Autodesk Inventor part; units mm, degrees
ref_plane "YZ Plane" through (0, 0, 0) normal (1, 0, 0) x (0, 1, 0)
ref_plane "XZ Plane" through (0, 0, 0) normal (0, 1, 0) x (-1, 0, 0)
ref_plane "XY Plane" through (0, 0, 0) normal (0, 0, 1) x (1, 0, 0)
sketch "Sketch1" plane through (0, 0, 0) normal (0, 0, 1) x (1, 0, 0)
  circle A0 centre (0, 0) radius 5
  circle A1 centre (0, 0) radius 2.5
  dimension "d0" = 10
  dimension "d1" = 5
extrude "Extrusion1" add sketch "Sketch1" along normal mid plane 4.2
sketch "Sketch2" plane through (0, 0, 2.1) normal (0, 0, 1) x (1, 0, 0)
  circle A0 centre (0, 0) radius 2.5
  circle A1 centre (0, 0) radius 5
  circle A2 centre (0, 0) radius 4.5
  circle A3 centre (0, 0) radius 4.1
  circle A4 centre (0, 0) radius 2.95
  circle A5 centre (0, 0) radius 3.35
  dimension "d4" = 0.5
  dimension "d5" = 0.4
  dimension "d6" = 0.75
  dimension "d7" = 0.4
extrude "Extrusion2" cut sketch "Sketch2" against normal blind 0.5 contours A2 | A5
fillet "Fillet1" radius 0.15 2 edges at (-4.1, 0, 2.1) (-3.35, 0, 2.1)
mirror "Mirror1" about plane through (0, 0, 0) normal (0, 0, 1) of "Extrusion2"
fillet "Fillet2" radius 0.15 2 edges at (-4.1, 0, -2.1) (-3.35, 0, -2.1)
properties part number "Mini Bearing" material "Steel"
Can you work these out from the model? Positions are in its coordinate system, mm. A direction names the side the tool comes from. Give positions to 0.01 mm unless a question says otherwise; leave off trailing zeros. Loops run counter-clockwise (first coordinate to the right, second up) from the corner with the lowest first, then second, coordinate; pieces in that order, holes last. Notation, with made-up numbers: (-32.75, -26.75) -> (-5.75, -26.75) arc R14 ccw to (-5.75, -7.75) -> close; hole circle Ø8 at (33.5, 14). An arc over 180 degrees is marked (long way). Return JSON: item names as keys, results as strings.
Q1. I want a section at A-A, the plane z = -0.45. List the corners of the cut face in (x, y) for me.
Checks:
{"outline": "circle Ø10 at (0, 0); hole circle Ø5 at (0, 0)"}
Q2. On a 3-axis mill with a long thin cutter (end or side, diameter ignored), from which of +Z, -Z, +X, -X, +Y, -Y can I reach the whole of each face in a straight line? I mean faces 1 (the face through (-0.54, -2.44, 0.03)), 2 (the face through (-0.534, 4.065, 1.777)), 3 (the face through (-1, -3, -1.6)). Say none if no direction works.
Checks:
{"face 1": "+Z, -Z", "face 2": "+Z", "face 3": "-Z"}
Q3. For pin 1 Ø1 at (x, z) = (-1, 1) entering from -Y; pin 2 Ø4.5 at (x, y) = (0, 0) entering from -Z, each with a flat end and sliding along its axis, tell me the tip position at first contact or that it passes through.
Checks:
{"pin 1": "stops at y = -4.97", "pin 2": "passes through"}
Q4. I need wall thicknesses on probe 1 along Y at (x, z) = (0, 1.8); probe 2 along X at (y, z) = (1.5, -1.7); probe 3 along Z at (x, y) = (-2.25, 3.5). Which ranges of each line are inside material? Lowest first, please.
Checks:
{"probe 1": "y = -5 to -4.5, -4.1 to -3.35, -2.95 to -2.5, 2.5 to 2.95, 3.35 to 4.1, 4.5 to 5", "probe 2": "x = -4.77 to -4.24, -3.82 to -3, -2.54 to -2, 2 to 2.54, 3 to 3.82, 4.24 to 4.77", "probe 3": "z = -1.6 to 1.6"}
